CAD build for the part. Positions are in the model's coordinates, mm. A direction names the side the tool comes from. Give positions to 0.01 mm unless a question says otherwise; leave off trailing zeros. Loops run counter-clockwise (first coordinate to the right, second up) from the corner with the lowest first, then second, coordinate; pieces in that order, holes last. Notation, with made-up numbers: M -14,-35 L 12,-35 A13 ccw 12,-23 Z; hole C 89.5,25.25 d4. An arc over 180 degrees is marked long. One line per question, with ' | ' between items.
```python
from build123d import *

# Parameters (mm, degrees)
F0_W     = 105
F0_H     = 65
F1_DEPTH = 50
F2_W     = 25
F2_H     = 35.092428
F2_H_2   = 36.408834
F3_DEPTH = 65
F5_DEPTH = 105


with BuildPart() as f1:
    # F0 (on Front) → F1 (new body)
    with BuildSketch(Plane.XZ):
        Rectangle(F0_W, F0_H)
    extrude(amount=-F1_DEPTH)

    # F2 (on face) → F3 (cut)
    with BuildSketch(Plane.XY.offset(32.5)):
        with Locations((40, 17.546214)):
            Rectangle(F2_W, F2_H)
        with Locations((-10, 18.204417)):
            Rectangle(F2_W, F2_H_2)
    extrude(amount=-F3_DEPTH, mode=Mode.SUBTRACT)

    # F4 (on face) → F5 (cut)
    with BuildSketch(Plane(origin=(-52.5, 0, 0), x_dir=(0, -1, 0), z_dir=(-1, 0, 0))):
        Polygon((0, 32.5), (-50, 32.5), (0, 0), align=None)
    extrude(amount=-F5_DEPTH, mode=Mode.SUBTRACT)


solid = f1.part
```
Item 1: Saw through at D-D on x = 24. Give the cut face in (y, z), and give its area (3 significant figures).
Conclusion:
outline: M 0,-32.5 L 50,-32.5 L 50,32.5 L 0,0 Z | area: 2,440 mm²
Item 2: Drill centre lines: line 1 along X through (y, z) = (21, -22.5); line 2 along X through (y, z) = (36, -0.5); line 3 along Y through (x, z) = (-1.5, -30). Where is each one in solid material? Low to high. Write a range as [from, to].
Conclusion:
line 1: [-52.5, -22.5], [2.5, 27.5] | line 2: [-52.5, -22.5], [2.5, 52.5] | line 3: [36.41, 50]
Item 3: Saw through at A-A on y = 3. Give the cut face in (x, z), and give its area (3 significant figures).
Conclusion:
outline: M -52.5,-32.5 L -22.5,-32.5 L -22.5,1.95 L -52.5,1.95 Z; M 2.5,-32.5 L 27.5,-32.5 L 27.5,1.95 L 2.5,1.95 Z | area: 1,890 mm²
Item 4: 3-axis set-ups, long thin cutter, end or side, ignore diameter. For faces 5 (the flat face through (27.5, 17, -11)), 6 (the flat face through (-10, 36.409, -4)), 7 (the flat face through (-1, 50, 0)): which of +Z, -Z, +X, -X, +Y, -Y reach the whole face in a straight line?
Conclusion:
face 5: +Z, -Z, +X, -Y | face 6: +Z, -Z, -Y | face 7: +Z, -Z, +X, -X, +Y
Item 5: Mould opens along X. For faces 1 (the flat face through (40, 35.092, -4)), 2 (the flat face through (2.5, 18, -10)), 3 (the flat face through (-52.5, 25, -8)), 4 (the flat face through (-22.5, 18, -10)) say: pulls with the +X half, pulls with the -X half, needs draft (parallel to the pull), parting line crosses it, or undercut.
Conclusion:
face 1: needs draft | face 2: undercut | face 3: pulls with the -X half | face 4: undercut
Item 6: Drop flat-ended pins along their axis: P1, Ø1.5, axis at y = 33, z = -21, coming from the +X side; P2, Ø20, axis at x = 43, z = -13, coming from the -Y side; P3, Ø3, axis at x = 10, y = 31, coming from the +Z side (3 decimals). Give the stop position or say it passes through.
Conclusion:
P1: x = 27.5 | P2: y = 35.09 | P3: z = 21.125
Item 7: Saw through at C-C on y = 12. Give the cut face in (x, z), and give its area (3 significant figures).
Conclusion:
outline: M -52.5,-32.5 L -22.5,-32.5 L -22.5,7.8 L -52.5,7.8 Z; M 2.5,-32.5 L 27.5,-32.5 L 27.5,7.8 L 2.5,7.8 Z | area: 2,220 mm²
Item 8: Saw through at B-B on z = 1.5. Give the cut face in (x, y), and give its area (3 significant figures).
Conclusion:
outline: M -52.5,2.31 L -22.5,2.31 L -22.5,36.41 L 2.5,36.41 L 2.5,2.31 L 27.5,2.31 L 27.5,35.09 L 52.5,35.09 L 52.5,50 L -52.5,50 Z | area: 3,340 mm²
